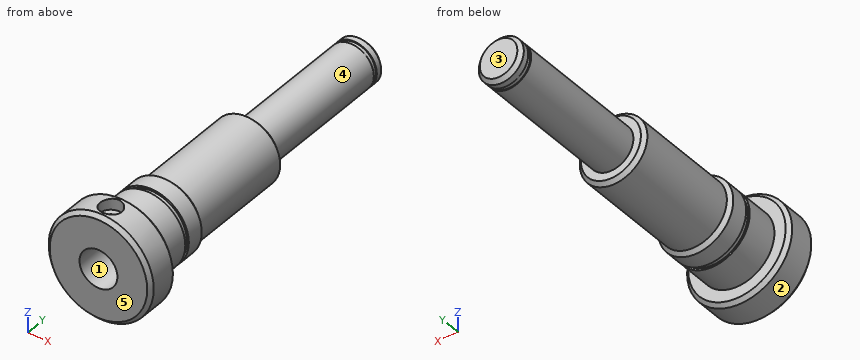
```python
from build123d import *

# Parameters (mm, degrees)
CHAMFER2_SIZE               = 1
CHAMFER7_SIZE               = 1
CHAMFER8_SIZE               = 1
CHAMFER9_SIZE               = 1
SKETCH2_R                   = 5.05
CUT_EXTRUDE1_DEPTH          = 20.5
SKETCH3_R                   = 2.9
CUT_EXTRUDE2_DEPTH          = 3
TAP_DRILL_FOR_M3_TAP1_D     = 2.5
TAP_DRILL_FOR_M3_TAP1_DEPTH = 8
TAP_DRILL_FOR_M3_TAP1_TIP   = 0.751075774


with BuildPart() as part:
    # Sketch1 → Revolve1 (revolve)
    with BuildSketch(Plane.XY, mode=Mode.PRIVATE) as revolve1_sk:
        Polygon((0, 0), (-10, 0), (-14, 0), (-14, 9), (-10, 9), (-10, 18), (-9.5, 18), (-9.5, 19.3), (-10, 19.3), (-10, 25), (-9, 25), (-9, 55), (-6, 55), (-6, 92.3), (-5.75, 92.3), (-5.75, 93.4), (-6, 93.4), (-6, 96), (0, 96), align=None)
    revolve(revolve1_sk.sketch.rotate(Axis((0, 0, 0), (0, 1, 0)), 180), axis=Axis((0, 0, 0), (0, 1, 0)))

    # Chamfer2
    chamfer2_edges = [part.edges().sort_by_distance(p)[0] for p in [
        (-6, 96, 0),
    ]]
    chamfer(chamfer2_edges, length=CHAMFER2_SIZE)

    # Chamfer7
    chamfer7_edges = [part.edges().sort_by_distance(p)[0] for p in [
        (-9, 55, 0),
    ]]
    chamfer(chamfer7_edges, length=CHAMFER7_SIZE)

    # Chamfer8
    chamfer8_edges = [part.edges().sort_by_distance(p)[0] for p in [
        (-10, 25, 0),
    ]]
    chamfer(chamfer8_edges, length=CHAMFER8_SIZE - 0.0001)  # a hair under: the kernel refuses the full size

    # Chamfer9
    chamfer9_edges = [part.edges().sort_by_distance(p)[0] for p in [
        (-14, 9, 0),
        (-14, 0, 0),
    ]]
    chamfer(chamfer9_edges, length=CHAMFER9_SIZE)

    # Sketch2 → Cut-Extrude1 (cut)
    with BuildSketch(Plane.XZ):
        Circle(SKETCH2_R)
    extrude(amount=-CUT_EXTRUDE1_DEPTH, mode=Mode.SUBTRACT)

    # Sketch3 → Cut-Extrude2 (cut)
    with BuildSketch(Plane.XY.offset(14)):
        with Locations((0, 4.5)):
            Circle(SKETCH3_R)
    extrude(amount=-CUT_EXTRUDE2_DEPTH, mode=Mode.SUBTRACT)

    # Tap Drill for M3 Tap1
    with Locations(Plane(origin=(0, 4.5, 11), x_dir=(1, 0, 0), z_dir=(0, 0, 1))):
        with Locations((0, 0)):
            Hole(TAP_DRILL_FOR_M3_TAP1_D / 2, depth=TAP_DRILL_FOR_M3_TAP1_DEPTH)
            with Locations((0, 0, -(TAP_DRILL_FOR_M3_TAP1_DEPTH + TAP_DRILL_FOR_M3_TAP1_TIP / 2))):  # 118° drill point
                Cone(0, TAP_DRILL_FOR_M3_TAP1_D / 2, TAP_DRILL_FOR_M3_TAP1_TIP, mode=Mode.SUBTRACT)


solid = part.part
```
Check sheet for the modelled part. Datum: model origin and axes. Units: mm. Face numbers are marked on the shaded views. A direction names the side the tool comes from. Coordinates: 2 decimals unless noted, no trailing zeros. Loops run counter-clockwise (first coordinate to the right, second up) from the corner with the lowest first, then second, coordinate; pieces in that order, holes last.
1) Sectioned sample at B-B (y = 75). Record the boundary of the cut face in (x, z).
2) Material ranges on probe 1 along Y at (x, z) = (0, 7.5); probe 2 along Z at (x, y) = (0, 4.5); probe 3 along Y at (x, z) = (0, 12.45), recorded low to high.
3) Sectioned sample at A-A (y = 4.5). Record the boundary of the cut face in (x, z).
4) Gauge pin test, flat ends, axial feed: pin 1 (12 mm diameter, centred on x = -6.5, y = 55.5, fed in from +Z); pin 2 (12 mm diameter, centred on y = 34, z = 6.5, fed in from +X); pin 3 (10 mm diameter, centred on x = 0.5, y = 72.5, fed in from +Z). Record the tip position at first contact, or that the pin passes through.
5) Access from +Z, -Z, +X, -X, +Y, -Y to the whole of each face (thin tool, end or side, straight path). Record for the marked faces 4 and 5.
6) Release check for a two-part mould opening along Z. For the marked faces 1, 2 and 3 record: released by +Z, released by -Z, zero draft, split by the parting line, or undercut.
Check sheet entries:
1. outline: circle Ø12 at (0, 0)
2. probe 1: y = 0 to 3.25, 5.75 to 55
2. probe 2: z = -14 to -5.05
2. probe 3: y = 0 to 1.6, 7.4 to 9
3. outline: (-2.9, 11) - (-2.9, 13.7) arc R14 ccw (long way) to (2.9, 13.7) - (2.9, 11) - (1.25, 11) - (1.25, 4.89) arc R5.05 cw (long way) to (-1.25, 4.89) - (-1.25, 11) - close
4. pin 1: stops at z = 8.97
4. pin 2: stops at x = 8.99
4. pin 3: stops at z = 6
5. face 4: +Y
5. face 5: +Z, -Z, +X, -X, -Y
6. face 1: undercut
6. face 2: split by the parting line
6. face 3: zero draft
